Part model, mm, in its own coordinate system. Give positions to 0.01 mm unless a question says otherwise; leave off trailing zeros. Write each loop counter-clockwise with the first axis right and the second up, starting at its lowest first coordinate (ties: lowest second). Pieces come first, ordered by that corner, then holes.
Autodesk Inventor part; units mm, degrees
ref_plane "YZ Plane" through (0, 0, 0) normal (1, 0, 0) x (0, 1, 0)
ref_plane "XZ Plane" through (0, 0, 0) normal (0, 1, 0) x (-1, 0, 0)
ref_plane "XY Plane" through (0, 0, 0) normal (0, 0, 1) x (1, 0, 0)
sketch "Sketch1" plane through (0, 0, 0) normal (0, 0, 1) x (1, 0, 0)
  line L0 (0, 0) -> (10, 0)
  line L1 (10, 0) -> (10, 8)
  line L2 (10, 8) -> (0, 8)
  line L3 (0, 8) -> (0, 0)
  dimension "d0" = 10
  dimension "d1" = 8
extrude "Extrusion1" add sketch "Sketch1" along normal blind 0.1
sketch "Sketch2" plane through (0, 0, 0) normal (0, -1, 0) x (1, 0, 0)
  circle A0 centre (5, 0.05) radius 0.225
  dimension "d4" = 0.45
extrude "Extrusion2" add sketch "Sketch2" against normal blind 8
sketch "Sketch3" plane through (0, 0, 0.1) normal (0, 0, 1) x (1, 0, 0)
  point P0 (1, 7)
  point P1 (1, 1)
hole "Hole1" at (1, 7, 0.1) at (1, 1, 0.1) direction (0, 0, -1) diameter 1.2 end through all
sketch "Sketch4" plane through (0, 0, 0.1) normal (0, 0, 1) x (1, 0, 0)
  point P0 (0, 0)
  point P1 (9, 7)
  point P2 (9, 1)
hole "Hole2" at (9, 7, 0.1) at (9, 1, 0.1) direction (0, 0, -1) diameter 1.2 end through all
sketch "Sketch5" plane through (0, 0, 0.1) normal (0, 0, 1) x (1, 0, 0)
  line L0 (4.7806, 0) -> (4.7806, 8)
  line L1 (4.7806, 0) -> (4.5306, 0)
  line L2 (4.5306, 0) -> (4.5306, 0.5)
  line L3 (4.5306, 0.5) -> (4.7806, 0.5)
  line L4 (4.7806, 0.5) -> (4.7806, 0)
  line L5 (4.5306, 1) -> (4.7806, 1)
  line L6 (4.7806, 1) -> (4.7806, 1.5)
  line L7 (4.7806, 1.5) -> (4.5306, 1.5)
  line L8 (4.5306, 1.5) -> (4.5306, 1)
  line L9 (4.7806, 2) -> (4.5306, 2)
  line L10 (4.5306, 2) -> (4.5306, 2.5)
  line L11 (4.5306, 2.5) -> (4.7806, 2.5)
  line L12 (4.7806, 2.5) -> (4.7806, 2)
  line L13 (4.7806, 3) -> (4.5306, 3)
  line L14 (4.5306, 3) -> (4.5306, 3.5)
  line L15 (4.5306, 3.5) -> (4.7806, 3.5)
  line L16 (4.7806, 3.5) -> (4.7806, 3)
  line L17 (4.7806, 4) -> (4.5306, 4)
  line L18 (4.5306, 4) -> (4.5306, 4.5)
  line L19 (4.5306, 4.5) -> (4.7806, 4.5)
  line L20 (4.7806, 4.5) -> (4.7806, 4)
  line L21 (4.7806, 5) -> (4.5306, 5)
  line L22 (4.5306, 5) -> (4.5306, 5.5)
  line L23 (4.5306, 5.5) -> (4.7806, 5.5)
  line L24 (4.7806, 5.5) -> (4.7806, 5)
  line L25 (4.7806, 6) -> (4.5306, 6)
  line L26 (4.5306, 6) -> (4.5306, 6.5)
  line L27 (4.5306, 6.5) -> (4.7806, 6.5)
  line L28 (4.7806, 6.5) -> (4.7806, 6)
  line L29 (4.7806, 7) -> (4.5306, 7)
  line L30 (4.5306, 7) -> (4.5306, 7.5)
  line L31 (4.5306, 7.5) -> (4.7806, 7.5)
  line L32 (4.7806, 7.5) -> (4.7806, 7)
  dimension "d21" = 0.25
  dimension "d22" = 0.5
  dimension "d23" = 0.5
  dimension "d24" = 0.5
  dimension "d25" = 0.5
  dimension "d26" = 0.5
  dimension "d27" = 0.5
  dimension "d28" = 0.5
  dimension "d29" = 0.5
extrude "Extrusion3" cut sketch "Sketch5" against normal blind 8
sketch "Sketch6" plane through (0, 0, 0.1) normal (0, 0, 1) x (1, 0, 0)
  line L0 (10, 8) -> (5.2194, 8)
  line L1 (5.2194, 0) -> (5.2194, 8)
  line L2 (5.2194, 0.5) -> (5.4694, 0.5)
  line L3 (5.4694, 0.5) -> (5.4694, 1)
  line L4 (5.4694, 1) -> (5.2194, 1)
  line L5 (5.2194, 1) -> (5.2194, 0.5)
  line L6 (5.2194, 1.5) -> (5.4694, 1.5)
  line L7 (5.4694, 1.5) -> (5.4694, 2)
  line L8 (5.4694, 2) -> (5.2194, 2)
  line L9 (5.2194, 2) -> (5.2194, 1.5)
  line L10 (5.2194, 2.5) -> (5.4694, 2.5)
  line L11 (5.4694, 2.5) -> (5.4694, 3)
  line L12 (5.4694, 3) -> (5.2194, 3)
  line L13 (5.2194, 3) -> (5.2194, 2.5)
  line L14 (5.2194, 3.5) -> (5.4694, 3.5)
  line L15 (5.4694, 3.5) -> (5.4694, 4)
  line L16 (5.4694, 4) -> (5.2194, 4)
  line L17 (5.2194, 4) -> (5.2194, 3.5)
  line L18 (5.2194, 4.5) -> (5.4694, 4.5)
  line L19 (5.4694, 4.5) -> (5.4694, 5)
  line L20 (5.4694, 5) -> (5.2194, 5)
  line L21 (5.2194, 5) -> (5.2194, 4.5)
  line L22 (5.2194, 5.5) -> (5.4694, 5.5)
  line L23 (5.4694, 5.5) -> (5.4694, 6)
  line L24 (5.4694, 6) -> (5.2194, 6)
  line L25 (5.2194, 6) -> (5.2194, 5.5)
  line L26 (5.2194, 6.5) -> (5.4694, 6.5)
  line L27 (5.4694, 6.5) -> (5.4694, 7)
  line L28 (5.4694, 7) -> (5.2194, 7)
  line L29 (5.2194, 7) -> (5.2194, 6.5)
  line L30 (5.2194, 7.5) -> (5.4694, 7.5)
  line L31 (5.4694, 7.5) -> (5.4694, 8)
  line L32 (5.4694, 8) -> (5.2194, 8)
  line L33 (5.2194, 8) -> (5.2194, 7.5)
  point P0 (0, 0)
  dimension "d32" = 0.25
  dimension "d33" = 0.5
  dimension "d36" = 0.5
  dimension "d37" = 0.5
  dimension "d38" = 0.5
  dimension "d39" = 0.5
  dimension "d40" = 0.5
  dimension "d41" = 0.5
extrude "Extrusion4" cut sketch "Sketch6" against normal blind 8
fillet "Fillet1" radius 0.5 4 edges at (0, 0, 0.05) (0, 8, 0.05) (10, 8, 0.05) (10, 0, 0.05)
properties part number "Scharnier"
1) Drill centre line: L1, parallel to X at y = 3.5, z = 0.2. Where is it in solid material? Low to high.
Check result:
L1: x = 4.83 to 5.17
2) Saw through at C-C (x = 7.25). Write the cut outline in (y, z), and give its area (3 significant figures).
Check result:
outline: (0, 0) - (8, 0) - (8, 0.1) - (0, 0.1) - close
area: 0.800 mm2
3) Flat gauge pins, fed straight in: P1, Ø1.1, axis at x = 1, y = 7, coming from the +Z side; P2, Ø2, axis at x = 2.5, y = 6, coming from the -Z side. Where does each tip first touch, or does it go through?
Check result:
P1: passes through
P2: stops at z = 0
4) Saw through at A-A (x = 1). Write the cut outline in (y, z).
Check result:
outline: (0, 0) - (0.4, 0) - (0.4, 0.1) - (0, 0.1) - close; (1.6, 0) - (6.4, 0) - (6.4, 0.1) - (1.6, 0.1) - close; (7.6, 0) - (8, 0) - (8, 0.1) - (7.6, 0.1) - close
